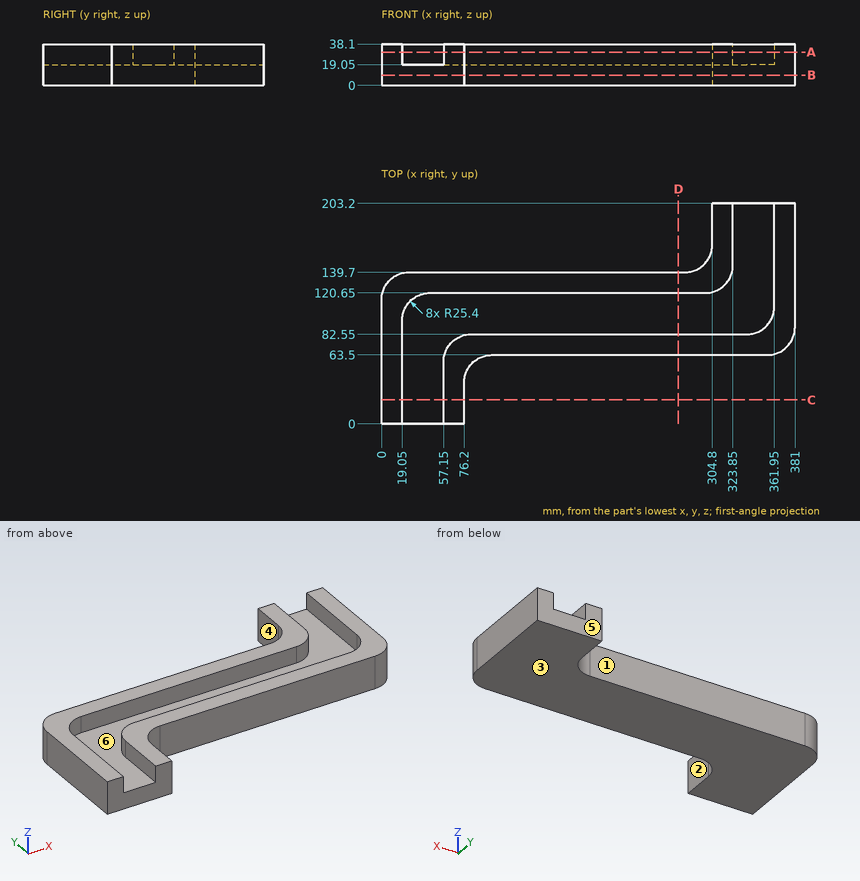
Source: three-view drawing plus pictorial views. Frame: mm from the lowest corner of the part. A direction names the side the tool comes from. Give positions to 0.01 mm unless a question says otherwise; leave off trailing zeros. Order: outer loops, then holes, each group sorted by start corner. A loop starts at its lowest first (then second) coordinate and runs counter-clockwise, first axis right, second up. Notation, with made-up numbers: (14, 23.5) - (58, 23.5) arc R13 cw to (58, 33.5) - close; hole circle Ø3 at (27, -28.5). An arc over 180 degrees is marked (long way). Put each result on its own line as item: value.
Item 1: Contact query for flat-ended pins moving along their axis: pin 1 (5.5 mm diameter, centred on y = 145, z = 27.5, fed in from -X); pin 2 (1 mm diameter, centred on x = 252, z = 15, fed in from +Y); pin 3 (6 mm diameter, centred on y = 84.5, z = 21.5, fed in from +X). Output: stop coordinate, or through.
Found:
pin 1: stops at x = 290.49
pin 2: stops at y = 139.7
pin 3: stops at x = 380.96
Item 2: Draft query along Y for the marked faces 4, 5 and 6. Return one class per face: +Y half, -Y half, draft (parallel to the pull), parting line (faces both ways), or undercut.
Found:
face 4: draft
face 5: +Y half
face 6: undercut
Item 3: Ray query, L1, parallel to Y at x = 191.5, z = 34.5; L2, parallel to X at y = 169, z = 25.5; L3, parallel to Y at x = 342, z = 18. Return the intervals inside material, ascending. Write a range as from..to.
Found:
L1: y = 63.5..82.55, 120.65..139.7
L2: x = 304.8..323.85, 361.95..381
L3: y = 63.5..203.2
Item 4: Section query D-D, the plane x = 273.5. Return loops of the section in (y, z), then the cut area to 3 significant figures.
Found:
outline: (63.5, 0) - (139.7, 0) - (139.7, 38.1) - (120.65, 38.1) - (120.65, 19.05) - (82.55, 19.05) - (82.55, 38.1) - (63.5, 38.1) - close
area: 2,180 mm^2
Item 5: Section query B-B, the plane z = 9.5. Return loops of the section in (x, y), then the cut area to 3 significant figures.
Found:
outline: (0, 0) - (76.2, 0) - (76.2, 38.1) arc R25.4 cw to (101.6, 63.5) - (355.6, 63.5) arc R25.4 ccw to (381, 88.9) - (381, 203.2) - (304.8, 203.2) - (304.8, 165.1) arc R25.4 cw to (279.4, 139.7) - (25.4, 139.7) arc R25.4 ccw to (0, 114.3) - close
area: 38,700 mm^2
Item 6: Access query for the marked faces 1, 2 and 3. Directions: +Z, -Z, +X, -X, +Y, -Y. A direction counts if a zero-diameter tool reaches every point of the face in a straight line with its end or side. Return the directions, or none.
Found:
face 1: +Z, -Z, -X, +Y
face 2: +Z, -Z, +X, -Y
face 3: -Z, +X, -X, +Y, -Y
Item 7: Section query C-C, the plane y = 22. Return loops of the section in (x, z), then the cut area to 3 significant figures.
Found:
outline: (0, 0) - (76.2, 0) - (76.2, 38.1) - (57.15, 38.1) - (57.15, 19.05) - (19.05, 19.05) - (19.05, 38.1) - (0, 38.1) - close
area: 2,180 mm^2
Item 8: Section query A-A, the plane z = 30.5. Return loops of the section in (x, y).
Found:
outline: (0, 0) - (19.05, 0) - (19.05, 95.25) arc R25.4 cw to (44.45, 120.65) - (298.45, 120.65) arc R25.4 ccw to (323.85, 146.05) - (323.85, 203.2) - (304.8, 203.2) - (304.8, 165.1) arc R25.4 cw to (279.4, 139.7) - (25.4, 139.7) arc R25.4 ccw to (0, 114.3) - close; (57.15, 0) - (76.2, 0) - (76.2, 38.1) arc R25.4 cw to (101.6, 63.5) - (355.6, 63.5) arc R25.4 ccw to (381, 88.9) - (381, 203.2) - (361.95, 203.2) - (361.95, 107.95) arc R25.4 cw to (336.55, 82.55) - (82.55, 82.55) arc R25.4 ccw to (57.15, 57.15) - close
